The model under review builds one solid part; all positions refer to its coordinate system, in mm. Face numbers are marked on the shaded views. A direction names the side the tool comes from. Coordinates: 2 decimals unless noted, no trailing zeros. Loops run counter-clockwise (first coordinate to the right, second up) from the corner with the lowest first, then second, coordinate; pieces in that order, holes last. Notation, with made-up numbers: M 16,-32 L 73,-32 A13 ccw 73,-7 Z; hole C 62.5,35.5 d6. An arc over 180 degrees is marked long. Return JSON: item names as keys, results as strings.
```python
from build123d import *

# Parameters (mm, degrees)
F0_R     = 21.5
F0_R_2   = 16.4
F1_DEPTH = 27.25
F0_R_3   = 32.5
F2_DEPTH = 1.5
F0_R_4   = 14.2
F3_DEPTH = 1
F5_DEPTH = 5
F6_R     = 0.75
F7_SIZE  = 0.99999
F8_DEPTH = 1


# Not quite as in the source:
# - a fillet or chamfer is up to 0.001 mm smaller than in the source, because OpenCascade refuses the exact size


with BuildPart() as f1:
    # F0 (on Top) → F1 (new body)
    with BuildSketch(Plane.XY):
        Circle(F0_R)
        Circle(F0_R_2, mode=Mode.SUBTRACT)
    extrude(amount=F1_DEPTH)

    # F0 (on Top) → F2 (join)
    with BuildSketch(Plane.XY):
        Circle(F0_R_3)
        Circle(F0_R, mode=Mode.SUBTRACT)
    extrude(amount=F2_DEPTH)

    # F0 (on Top) → F3 (join)
    with BuildSketch(Plane.XY):
        Circle(F0_R_2)
        Circle(F0_R_4, mode=Mode.SUBTRACT)
    extrude(amount=F3_DEPTH)

    # F4 (on face) → F5 (cut)
    with BuildSketch(Plane.XY.offset(27.25)):
        with BuildLine():
            ThreePointArc((-1.4988901219, 19.4423076923), (0, 18), (1.4988901219, 19.4423076923))
            ThreePointArc((1.4988901219, 19.4423076923), (0, 19.5), (-1.4988901219, 19.4423076923))
        make_face()
        with BuildLine():
            ThreePointArc((-1.4988901219, 19.4423076923), (0, 19.5), (1.4988901219, 19.4423076923))
            ThreePointArc((1.4988901219, 19.4423076923), (1.4997225048, 19.4711485087), (1.5, 19.5))
            ThreePointArc((1.5, 19.5), (-0.0288514913, 20.9997225048), (-1.4988901219, 19.4423076923))
        make_face()
        with BuildLine():
            ThreePointArc((18.3874953738, -9.75), (18.171867416, -8.9751526232), (17.5869774307, -8.4230769231))
            ThreePointArc((17.5869774307, -8.4230769231), (16.8874953738, -9.75), (16.0880873088, -11.0192307692))
            ThreePointArc((16.0880873088, -11.0192307692), (17.6123705018, -11.0632235334), (18.3874953738, -9.75))
        make_face()
        with BuildLine():
            ThreePointArc((16.0880873088, -11.0192307692), (16.8874953738, -9.75), (17.5869774307, -8.4230769231))
            ThreePointArc((17.5869774307, -8.4230769231), (15.5884572681, -9), (16.0880873088, -11.0192307692))
        make_face()
        with BuildLine():
            ThreePointArc((-15.3874953738, -9.75), (-16.112647997, -8.4656279578), (-17.5869774307, -8.4230769231))
            ThreePointArc((-17.5869774307, -8.4230769231), (-16.8874953738, -9.75), (-16.0880873088, -11.0192307692))
            ThreePointArc((-16.0880873088, -11.0192307692), (-15.5742718404, -10.474875128), (-15.3874953738, -9.75))
        make_face()
        with BuildLine():
            ThreePointArc((-16.0880873088, -11.0192307692), (-16.8874953738, -9.75), (-17.5869774307, -8.4230769231))
            ThreePointArc((-17.5869774307, -8.4230769231), (-18.1865334795, -10.5), (-16.0880873088, -11.0192307692))
        make_face()
    extrude(amount=-F5_DEPTH, mode=Mode.SUBTRACT)

    # F6
    f6_edges = [f1.edges().sort_by_distance(p)[0] for p in [
        (-32.5, 0, 0),
    ]]
    fillet(f6_edges, radius=F6_R)

    # F7 (size 1 in the source; OpenCascade refuses exactly that, so slightly less here)
    f7_edges = [f1.edges().sort_by_distance(p)[0] for p in [
        (-14.2, 0, 0),
    ]]
    chamfer(f7_edges, length=F7_SIZE)

    # F8 (add): a face of the model
    f8_faces = [f1.faces().sort_by_distance(p)[0] for p in [
        (-15.9361379515, 0, 1),
    ]]
    extrude(f8_faces, amount=F8_DEPTH)


solid = f1.part
```
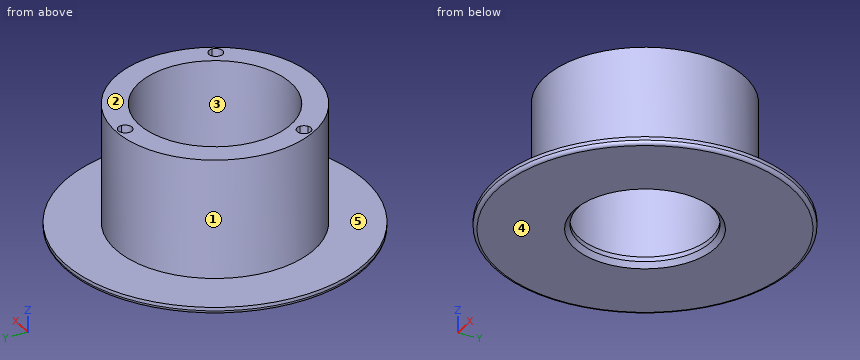
1. Add section B-B on x = 0. Give the boundary of the cut face in (y, z), plus the area to 3 significant figures.
Check values:
{"outline": "M -32.5,0.75 A0.75 ccw -31.75,0 L -15.2,0 L -14.2,1 L -14.2,2 L -16.4,2 L -16.4,27.25 L -21.5,27.25 L -21.5,1.5 L -32.5,1.5 Z; M 14.2,1 L 15.2,0 L 31.75,0 A0.75 ccw 32.5,0.75 L 32.5,1.5 L 21.5,1.5 L 21.5,27.25 L 21,27.25 L 21,22.25 L 18,22.25 L 18,27.25 L 16.4,27.25 L 16.4,2 L 14.2,2 Z", "area": "304 mm²"}
2. Add section A-A on y = 0. Give the boundary of the cut face in (x, z), plus the area to 3 significant figures.
Check values:
{"outline": "M -32.5,0.75 A0.75 ccw -31.75,0 L -15.2,0 L -14.2,1 L -14.2,2 L -16.4,2 L -16.4,27.25 L -21.5,27.25 L -21.5,1.5 L -32.5,1.5 Z; M 14.2,1 L 15.2,0 L 31.75,0 A0.75 ccw 32.5,0.75 L 32.5,1.5 L 21.5,1.5 L 21.5,27.25 L 16.4,27.25 L 16.4,2 L 14.2,2 Z", "area": "319 mm²"}
3. The part is to be moulded in two halves that separate along X. For the marked faces 1, 2 and 3, say which applies: released by +X, released by -X, zero draft, split by the parting line, or undercut.
Check values:
{"face 1": "split by the parting line", "face 2": "zero draft", "face 3": "undercut"}
4. Insertion check: pin 1 Ø3 at (x, z) = (10, 9) entering from +Y; pin 2 Ø0.9 at (x, y) = (-0.5, 19) entering from +Z; pin 3 Ø1 at (y, z) = (6.5, 9.5) entering from +X; pin 4 Ø1.5 at (x, y) = (-16.5, -10.5) entering from +Z. Each pin has a flat end and moves straight along its axis. Give the tip position at first contact, or say it passes through.
Check values:
{"pin 1": "y = 19.75", "pin 2": "z = 22.25", "pin 3": "x = 20.65", "pin 4": "z = 27.25"}
5. Machinability: for the marked faces 4 and 5, which of the approach directions +Z, -Z, +X, -X, +Y, -Y give a long, thin tool a straight path to every point of the face, cutting with its end or side? Answer none if there is none.
Check values:
{"face 4": "-Z, +X, -X, +Y, -Y", "face 5": "+Z"}
6. Add section C-C on z = 14.75. Give the boundary of the cut face in (x, y).
Check values:
{"outline": "C 0,0 d43; hole C 0,0 d32.8"}
7. To check wall thickness, follow line 1 (Y direction, x = 0, z = 11); line 2 (Z direction, x = -21, y = -20); line 3 (Y direction, x = 9, z = 16.5). State the ranges of each line that lie inside material, in increasing order.
Check values:
{"line 1": "-21.5 to -16.4, 16.4 to 21.5", "line 2": "0 to 1.5", "line 3": "-19.53 to -13.71, 13.71 to 19.53"}
